```python
from build123d import *

# Parameters (mm, degrees)
SM_BASE_FLANGE_1_DEPTH = 1
OTHER_START            = 15
OTHER_1_DEPTH          = 40
OTHER_1_2_DEPTH        = 10
OTHER_START_2          = 45
OTHER_1_3_DEPTH        = 10
HOLE_WIZARD_M12_1_D    = 4
FILLET_1_R             = 5
FILLET_2_R             = 0.25


# Read off the part's stored shape, not the designer's step: 햄1
# Sheet-metal steps are written as plain solids
with BuildPart() as part:
    # Sketch 1 → 베이스-플랜지1 (new body)
    with BuildSketch(Plane.XY):
        Polygon((0, 0), (0, 20), (15, 20), (15, 25), (25, 25), (25, 20), (45, 20), (45, 25), (55, 25), (55, 20), (70, 20), (70, 0), align=None)
    extrude(amount=-SM_BASE_FLANGE_1_DEPTH)

    # Other 1 outline → Other 1 (cut)
    with BuildSketch(Plane.YZ.offset(OTHER_START)):
        with BuildLine():
            Line((25, 0), (24.732050807, 0))
            ThreePointArc((24.732050807, 0), (24, -0.732050808), (23, -1))
            Line((23, -1), (25, -1))
            Line((25, -1), (25, 0))
        make_face()
    extrude(amount=OTHER_1_DEPTH, mode=Mode.SUBTRACT)

    # Other 1 2 outline → Other 1 2 (add)
    with BuildSketch(Plane.YZ.offset(OTHER_START)):
        with BuildLine():
            Line((21.030384494, 0.652703645), (22.015192247, 0.826351822))
            ThreePointArc((22.015192247, 0.826351822), (23.64278761, 1.766044443), (23, 0))
            Line((23, 0), (24.732050807, 0))
            ThreePointArc((24.732050807, 0), (23.347296355, 2.969615506), (21.030384494, 0.652703645))
        make_face()
    extrude(amount=OTHER_1_2_DEPTH)

    # Other 1 3 outline → Other 1 3 (add)
    with BuildSketch(Plane.YZ.offset(OTHER_START_2)):
        with BuildLine():
            Line((21.030384494, 0.652703645), (22.015192247, 0.826351822))
            ThreePointArc((22.015192247, 0.826351822), (23.64278761, 1.766044443), (23, 0))
            Line((23, 0), (24.732050807, 0))
            ThreePointArc((24.732050807, 0), (23.347296355, 2.969615506), (21.030384494, 0.652703645))
        make_face()
    extrude(amount=OTHER_1_3_DEPTH)

    # M12 여유 구멍1 (through all)
    with Locations(Plane(origin=(15, 10, 0), x_dir=(1, 0, 0), z_dir=(0, 0, 1))):
        with Locations((0, 0), (20, 0), (40, 0)):
            Hole(HOLE_WIZARD_M12_1_D / 2)

    # 필렛1
    fillet_1_edges = [part.edges().sort_by_distance(p)[0] for p in [
        (0, 0, -0.5),
        (70, 0, -0.5),
    ]]
    fillet(fillet_1_edges, radius=FILLET_1_R)

    # 필렛2
    fillet_2_edges = [part.edges().sort_by_distance(p)[0] for p in [
        (0, 20, -0.5),
        (15, 20, -0.5),
        (25, 20, -0.5),
        (45, 20, -0.5),
        (55, 20, -0.5),
        (70, 20, -0.5),
    ]]
    fillet(fillet_2_edges, radius=FILLET_2_R)


solid = part.part
```
Could you check a few things on this model? Use its own coordinates, in mm. A direction names the side the tool comes from. Coordinates: 2 decimals unless noted, no trailing zeros. Write each loop counter-clockwise with the first axis right and the second up, starting at its lowest first coordinate (ties: lowest second). Pieces come first, ordered by that corner, then holes. Notation, with made-up numbers: (87, 20) -> (95, 20) arc R21 cw to (95, 35) -> close; hole circle Ø5 at (16, 72). An arc over 180 degrees is marked (long way). One line per question, with ' | ' between items. Start each with the question number.
1. If we section it at B-B (x = 10.5): Please give me the cut outline in (y, z).
2. Will these pins go through, and if not, where does the flat tip stop? P1, Ø0.5, axis at x = 60, z = -0.5, coming from the +Y side; P2, Ø2, axis at y = 22, z = 1.5, coming from the +X side; P3, Ø1.2, axis at y = 21.5, z = 1, coming from the -X side.
3. If we section it at A-A (y = 9): Please give me the cut outline in (x, z).
4. For faces 4 (the face through (68.57, 1.5, -0.51)), 5 (the face through (45, 24, 0)), 6 (the face through (55, 24, 0)), which set-ups out of +Z, -Z, +X, -X, +Y, -Y let a thin tool reach every point of the face, with its end or its side?
5. Please list where these lines run through material, in increasing order: line 1 along Z through (x, y) = (52, 23); line 2 along X through (y, z) = (21.75, 1.65); line 3 along X through (y, z) = (11.5, -0.45).
6. If we section it at C-C (y = 13.5): Please give me the cut outline in (x, z), and give its area (3 significant figures).
7. Thinking about a two-plate mould opening in Y: for faces 1 (the face through (15.26, 11.983, -0.507)), 2 (the face through (15, 24, 0)), 3 (the face through (1.5, 1.43, -0.51)), which applies, pulls with the +Y half, pulls with the -Y half, needs draft (parallel to the pull), parting line crosses it, or undercut?
Return value:
1) outline: (0, -1) -> (20, -1) -> (20, 0) -> (0, 0) -> close
2) P1: stops at y = 20 | P2: stops at x = 55 | P3: stops at x = 15
3) outline: (0, -1) -> (13.27, -1) -> (13.27, 0) -> (0, 0) -> close; (16.73, -1) -> (33.27, -1) -> (33.27, 0) -> (16.73, 0) -> close; (36.73, -1) -> (53.27, -1) -> (53.27, 0) -> (36.73, 0) -> close; (56.73, -1) -> (70, -1) -> (70, 0) -> (56.73, 0) -> close
4) face 4: +Z, -Z, +X, -Y | face 5: +Z, -Z, +Y | face 6: +Z, -Z, +X, +Y
5) line 1: z = -1 to 0, 2 to 3 | line 2: x = 15 to 25, 45 to 55 | line 3: x = 0 to 13.68, 16.32 to 33.68, 36.32 to 53.68, 56.32 to 70
6) outline: (0, -1) -> (70, -1) -> (70, 0) -> (0, 0) -> close | area: 70.0 mm²
7) face 1: undercut | face 2: needs draft | face 3: pulls with the -Y half
